Build history of the part. All positions in model axes, mm. Face numbers are marked on the shaded views. A direction names the side the tool comes from. Round coordinates to 2 decimals unless told otherwise and drop trailing zeros. Loops run counter-clockwise (first coordinate to the right, second up) from the corner with the lowest first, then second, coordinate; pieces in that order, holes last. Notation, with made-up numbers: (-13.75, 62.5) - (15.25, 62.5) arc R25 cw to (15.25, 91.5) - close; hole circle Ø10 at (-13.75, -25). An arc over 180 degrees is marked (long way). Use one line per item in the form item = value. Start each with the question number.
Q1. Saw through at B-B (x = 29.5). Give the cut face in (y, z), then the cut area to 3 significant figures.
Q2. 3-axis set-ups, long thin cutter, end or side, ignore diameter. For the marked faces 1, 2 and 3: which of +Z, -Z, +X, -X, +Y, -Y reach the whole face in a straight line?
Q3. Saw through at D-D (x = -20.5). Give the cut face in (y, z), then the cut area to 3 significant figures.
Q4. Mould opens along Y. For the marked faces 4, 5 and 6 say: released by +Y, released by -Y, zero draft, split by the parting line, or undercut.
Q5. Saw through at C-C (z = -13.5). Count the separate pieces of the cut face and the enclosed holes in it, then the cut area to 3 significant figures.
Q6. Pin check, flat tips, straight feed: pin 1 (12 mm diameter, centred on x = 14.5, y = 6.5, fed in from -Z); pin 2 (1.5 mm diameter, centred on y = 8, z = -1.5, fed in from -X); pin 3 (14.5 mm diameter, centred on x = 1.5, y = -0.5, fed in from -Z); pin 4 (13 mm diameter, centred on x = 29.5, z = -10, fed in from -Y). Stop position of each tip, or through.
Q7. Drill centre lines: line 1 (Z direction, x = -29, y = 13); line 2 (Y direction, x = 0, z = 2.4); line 3 (X direction, y = 12, z = -11.5). Where is each one in solid material? Low to high.
```python
from build123d import *
from OCP.BRepFilletAPI import BRepFilletAPI_MakeChamfer
from build123d.topology import SkipClean

# Parameters (mm, degrees)
SKETCH1_W                 = 85
SKETCH1_H                 = 30
SKETCH1_R                 = 3.25
BOSS_EXTRUDE1_DEPTH       = 5
SKETCH3_R                 = 7.25
BOSS_EXTRUDE2_DEPTH       = 6
CHAMFER2_SIZE             = 5
CHAMFER2_SIZE2            = 5.261204957
FILLET1_R                 = 5
CHAMFER2_OF_MIRROR1_SIZE  = 5
CHAMFER2_OF_MIRROR1_SIZE2 = 5.261204957
FILLET1_OF_MIRROR1_R      = 5
BOSS_EXTRUDE3_START       = 5
SKETCH5_R                 = 6.5
SKETCH5_R_2               = 3.25
BOSS_EXTRUDE3_DEPTH       = 5
CHAMFER1_SIZE             = 5
CHAMFER3_SIZE             = 1


with BuildPart() as part:
    # Sketch1 → Boss-Extrude1 (new body)
    with BuildSketch(Plane.XY):
        Rectangle(SKETCH1_W, SKETCH1_H)
        Circle(SKETCH1_R, mode=Mode.SUBTRACT)
    extrude(amount=BOSS_EXTRUDE1_DEPTH)

    # Sketch3 → Boss-Extrude2 (add)
    # profile 1 of 2: a face of its own
    with BuildSketch(Plane(origin=(0, 15, 0), x_dir=(1, 0, 0), z_dir=(0, 1, 0))):
        with BuildLine():
            Line((42.5, 0), (41.985306827, 10.605898875))
            ThreePointArc((41.985306827, 10.605898875), (29.5, 22.5), (17.014693173, 10.605898875))
            Line((17.014693173, 10.605898875), (16.5, 0))
            Line((16.5, 0), (42.5, 0))
        make_face()
        with Locations(Location((29.5, 10, 0), (0, 0, 270))):
            Circle(SKETCH3_R, mode=Mode.SUBTRACT)
    # profile 2 of 2: a face of its own
    with BuildSketch(Plane(origin=(0, 15, 0), x_dir=(1, 0, 0), z_dir=(0, 1, 0))):
        with BuildLine():
            Line((-42.5, 0), (-41.985306827, 10.605898875))
            ThreePointArc((-41.985306827, 10.605898875), (-29.5, 22.5), (-17.014693173, 10.605898875))
            Line((-17.014693173, 10.605898875), (-16.5, 0))
            Line((-16.5, 0), (-42.5, 0))
        make_face()
        with Locations(Location((-29.5, 10, 0), (0, 0, 270))):
            Circle(SKETCH3_R, mode=Mode.SUBTRACT)
    boss_extrude2 = extrude(amount=-BOSS_EXTRUDE2_DEPTH)

    # Chamfer2: one chamfer whose edges measure the first distance from different faces: ONE call of the kernel's chamfer builder (chamfer() names one face for all edges)
    chamfer2_edges_1 = [part.edges().sort_by_distance(p)[0] for p in [
        (16.5, 12, 0),
    ]]
    chamfer2_side_1 = [part.faces().sort_by_distance(p)[0] for p in [
        (-41.598612181, -3, 0),
    ]]
    chamfer2_edges_2 = [part.edges().sort_by_distance(p)[0] for p in [
        (-16.5, 12, 0),
    ]]
    chamfer2_side_2 = [part.faces().sort_by_distance(p)[0] for p in [
        (-16.757346587, 12, -5.302949437),
    ]]
    chamfer2 = BRepFilletAPI_MakeChamfer(part.part.solid().wrapped)
    for e in chamfer2_edges_1:
        chamfer2.Add(CHAMFER2_SIZE, CHAMFER2_SIZE2, e.wrapped, chamfer2_side_1[0].wrapped)  # the first distance lies on this face
    for e in chamfer2_edges_2:
        chamfer2.Add(CHAMFER2_SIZE, CHAMFER2_SIZE2, e.wrapped, chamfer2_side_2[0].wrapped)  # the first distance lies on this face
    add(Compound.cast(chamfer2.Shape()), mode=Mode.REPLACE)

    # Fillet1
    fillet1_edges = [part.edges().sort_by_distance(p)[0] for p in [
        (11.5, 12, 0),
        (-11.238795043, 12, 0),
        (-16.74235955, 12, -4.994122731),
        (16.755020653, 12, -5.255020653),
    ]]
    fillet(fillet1_edges, radius=FILLET1_R)

    # Mirror1: Boss-Extrude2 across plane
    add(boss_extrude2.mirror(Plane.ZX))

    # Chamfer2 of Mirror1: one chamfer whose edges measure the first distance from different faces: ONE call of the kernel's chamfer builder (chamfer() names one face for all edges)
    chamfer2_of_mirror1_edges_1 = [part.edges().sort_by_distance(p)[0] for p in [
        (16.5, -12, 0),
    ]]
    chamfer2_of_mirror1_side_1 = [part.faces().sort_by_distance(p)[0] for p in [
        (-41.598612181, 3, 0),
    ]]
    chamfer2_of_mirror1_edges_2 = [part.edges().sort_by_distance(p)[0] for p in [
        (-16.5, -12, 0),
    ]]
    chamfer2_of_mirror1_side_2 = [part.faces().sort_by_distance(p)[0] for p in [
        (-16.757346587, -12, -5.302949437),
    ]]
    chamfer2_of_mirror1 = BRepFilletAPI_MakeChamfer(part.part.solid().wrapped)
    for e in chamfer2_of_mirror1_edges_1:
        chamfer2_of_mirror1.Add(CHAMFER2_OF_MIRROR1_SIZE, CHAMFER2_OF_MIRROR1_SIZE2, e.wrapped, chamfer2_of_mirror1_side_1[0].wrapped)  # the first distance lies on this face
    for e in chamfer2_of_mirror1_edges_2:
        chamfer2_of_mirror1.Add(CHAMFER2_OF_MIRROR1_SIZE, CHAMFER2_OF_MIRROR1_SIZE2, e.wrapped, chamfer2_of_mirror1_side_2[0].wrapped)  # the first distance lies on this face
    add(Compound.cast(chamfer2_of_mirror1.Shape()), mode=Mode.REPLACE)

    # Fillet1 of Mirror1
    fillet1_of_mirror1_edges = [part.edges().sort_by_distance(p)[0] for p in [
        (11.5, -12, 0),
        (-11.238795043, -12, 0),
        (-16.74235955, -12, -4.994122731),
        (16.755020653, -12, -5.255020653),
    ]]
    fillet(fillet1_of_mirror1_edges, radius=FILLET1_OF_MIRROR1_R)

    # Sketch5 → Boss-Extrude3 (add)
    with SkipClean():  # the faces are left unmerged after this step: merging them gives an invalid solid
        with BuildSketch(Plane(origin=(0, 0, 0), x_dir=(-1, 0, 0), z_dir=(0, 0, -1)).offset(BOSS_EXTRUDE3_START)):
            Circle(SKETCH5_R)
            Circle(SKETCH5_R_2, mode=Mode.SUBTRACT)
        extrude(amount=-BOSS_EXTRUDE3_DEPTH)

    # Chamfer1
    chamfer1_edges = [part.edges().sort_by_distance(p)[0] for p in [
        (6.5, 0, 0),
    ]]
    chamfer(chamfer1_edges, length=CHAMFER1_SIZE - 0.0001)  # a hair under: the kernel refuses the full size

    # Chamfer3
    chamfer3_edges = [part.edges().sort_by_distance(p)[0] for p in [
        (-42.5, 0, 5),
        (-3.25, 0, 5),
        (0, -15, 5),
        (42.5, 0, 5),
        (0, 15, 5),
    ]]
    chamfer(chamfer3_edges, length=CHAMFER3_SIZE)


solid = part.part
```
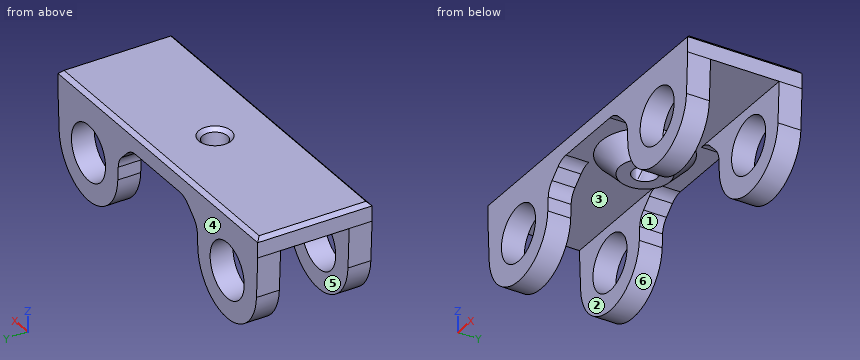
Report:
q1.outline = (-15, -22.5) - (-9, -22.5) - (-9, -17.25) - (-15, -17.25) - close; (-15, -2.75) - (-9, -2.75) - (-9, 0) - (9, 0) - (9, -2.75) - (15, -2.75) - (15, 4) - (14, 5) - (-14, 5) - (-15, 4) - close; (9, -22.5) - (15, -22.5) - (15, -17.25) - (9, -17.25) - close
q1.area = 245 mm²
q2.face_1 = -Z, +Y, -Y
q2.face_2 = -Z, -X
q2.face_3 = -Z
q3.outline = (-15, -18.67) - (-9, -18.67) - (-9, 0) - (9, 0) - (9, -18.67) - (15, -18.67) - (15, 4) - (14, 5) - (-14, 5) - (-15, 4) - close
q3.area = 373 mm²
q4.face_4 = released by +Y
q4.face_5 = undercut
q4.face_6 = zero draft
q5.separate_pieces = 8
q5.enclosed_holes = 0
q5.area = 271 mm²
q6.pin_1 = -18.07
q6.pin_2 = -7.44
q6.pin_3 = -5
q6.pin_4 = through
q7.line_1 = -22.49 to -17.23, -2.77 to 5
q7.line_2 = -15 to -3.25, 3.25 to 15
q7.line_3 = -41.91 to -36.59, -22.41 to -17.09, 17.09 to 22.41, 36.59 to 41.91
